```python
from build123d import *

# Parameters (mm, degrees)
BOSS_EXTRUDE1_DEPTH = 6
SKETCH2_R           = 1.8
CUT_EXTRUDE1_DEPTH  = 6
CIRPATTERN1_COUNT   = 4
SKETCH3_R           = 3
CUT_EXTRUDE2_DEPTH  = 7
SKETCH4_R           = 1
CUT_EXTRUDE3_DEPTH  = 10
CIRPATTERN2_COUNT   = 4


with BuildPart() as part:
    # Sketch1 → Boss-Extrude1 (new body)
    with BuildSketch(Plane.XY):
        Polygon((3, -30), (-3, -30), (-3, -17), (-17, -3), (-30, -3), (-30, 3), (-17, 3), (-3, 17), (-3, 30), (3, 30), (3, 17), (17, 3), (30, 3), (30, -3), (17, -3), (3, -17), align=None)
    extrude(amount=BOSS_EXTRUDE1_DEPTH)

    # Sketch2 → Cut-Extrude1 (cut)
    with BuildSketch(Plane(origin=(3, 0, 0), x_dir=(0, 0, -1), z_dir=(1, 0, 0))):
        with Locations((-3, 26.5)):
            Circle(SKETCH2_R)
    cut_extrude1 = extrude(amount=-CUT_EXTRUDE1_DEPTH, mode=Mode.SUBTRACT)

    # CirPattern1: Cut-Extrude1 ×4 about axis
    cirpattern1_axis = Axis((0, 0, 0), (0, 0, 1))
    for i in range(1, CIRPATTERN1_COUNT):
        add(cut_extrude1.rotate(cirpattern1_axis, i * 360 / CIRPATTERN1_COUNT), mode=Mode.SUBTRACT)

    # Sketch3 → Cut-Extrude2 (cut, through all)
    with BuildSketch(Plane.XY.offset(6)):
        Circle(SKETCH3_R)
    extrude(amount=-CUT_EXTRUDE2_DEPTH, mode=Mode.SUBTRACT)

    # Sketch4 → Cut-Extrude3 (cut)
    with BuildSketch(Plane.XY.offset(6)):
        with Locations((0, 10)):
            Circle(SKETCH4_R)
    cut_extrude3 = extrude(amount=-CUT_EXTRUDE3_DEPTH, mode=Mode.SUBTRACT)

    # CirPattern2: Cut-Extrude3 ×4 about axis
    cirpattern2_axis = Axis((0, 0, 0), (0, 0, 1))
    for i in range(1, CIRPATTERN2_COUNT):
        add(cut_extrude3.rotate(cirpattern2_axis, i * 360 / CIRPATTERN2_COUNT), mode=Mode.SUBTRACT)


solid = part.part
```
Work out the finished part from the listing and answer in its coordinate system (mm). A direction names the side the tool comes from. Coordinates: 2 decimals unless noted, no trailing zeros. Loops run counter-clockwise (first coordinate to the right, second up) from the corner with the lowest first, then second, coordinate; pieces in that order, holes last. Notation, with made-up numbers: (68.5, 8.5) - (99.5, 8.5) arc R26 ccw to (99.5, 36.5) - close; hole circle Ø7 at (22, 51). An arc over 180 degrees is marked (long way). Use a Markdown table: item, result.
Item 1: Find section C-C, the plane x = -7.5. Determine the outline of the cut face in (y, z), and give its area (3 significant figures).
Evaluation:
| item | result |
|---|---|
| outline | (-12.5, 0) - (12.5, 0) - (12.5, 6) - (-12.5, 6) - close |
| area | 150 mm2 |
Item 2: Find section D-D, the plane y = -16. Determine the outline of the cut face in (x, z).
Evaluation:
| item | result |
|---|---|
| outline | (-4, 0) - (4, 0) - (4, 6) - (-4, 6) - close |
Item 3: The mould has two halves that part along Z. Classify faces 1 (the cylindrical face through (-28.285, 0.042, 3.234)), 2 (the flat face through (2.4, -2.1, 6)), 3 (the flat face through (30, 0, 3)): +Z half, -Z half, draft (parallel to the pull), parting line (faces both ways), or undercut.
Evaluation:
| item | result |
|---|---|
| face 1 | undercut |
| face 2 | +Z half |
| face 3 | draft |
Item 4: Find section B-B, the plane z = 3. State how many separate pieces and enclosed holes the cut face has, and give its area (3 significant figures).
Evaluation:
| item | result |
|---|---|
| separate pieces | 5 |
| enclosed holes | 5 |
| area | 949 mm2 |
Item 5: For faces 4 (the flat face through (23, 3, 3)), 5 (the flat face through (-24, 3, 3)), 6 (the flat face through (-3, -24, 3)), 7 (the flat face through (3, -23, 3)), determine the directions among +Z, -Z, +X, -X, +Y, -Y from which every point of the face is accessible in a straight line to the end or side of a thin tool.
Evaluation:
| item | result |
|---|---|
| face 4 | +Z, -Z, +X, +Y |
| face 5 | +Z, -Z, -X, +Y |
| face 6 | +Z, -Z, -X, -Y |
| face 7 | +Z, -Z, +X, -Y |
Item 6: Consider probe 1 along Y at (x, z) = (-1.4, 3); probe 2 along Y at (x, z) = (18, 0.6). Determine where each line is inside the solid, lowest interval first. Write a range as from..to.
Evaluation:
| item | result |
|---|---|
| probe 1 | y = -30..-28.3, -24.7..-2.65, 2.65..24.7, 28.3..30 |
| probe 2 | y = -3..3 |
Item 7: Find section A-A, the plane y = 10. Determine the outline of the cut face in (x, z).
Evaluation:
| item | result |
|---|---|
| outline | (-10, 0) - (-1, 0) - (-1, 6) - (-10, 6) - close; (1, 0) - (10, 0) - (10, 6) - (1, 6) - close |
Item 8: Given pin 1 Ø1.8 at (y, z) = (-25.5, 2) entering from +X; pin 2 Ø1 at (x, z) = (-6, 2) entering from +Y; pin 3 Ø2 at (x, z) = (-21, 2) entering from -Y, each flat-ended and moving along its own axis, determine where each tip first touches the part or whether it passes through.
Evaluation:
| item | result |
|---|---|
| pin 1 | stops at x = 3 |
| pin 2 | stops at y = 14.5 |
| pin 3 | stops at y = -3 |
